```python
from build123d import *

# Parameters (mm, degrees)
CYLINDER004_R           = 5.625
CYLINDER004_DEPTH       = 20
ARRAY_COUNT             = 5
ARRAY_PLACEMENT_ANGLE   = 127.662
CYLINDER003_R           = 1.5
CYLINDER003_DEPTH       = 20
CYLINDER003_PITCH_ANGLE = 90
CYLINDER002_R           = 2.75
CYLINDER002_DEPTH       = 12
BOX_W                   = 3.25
BOX_H                   = 12
BOX_DEPTH               = 12
CYLINDER005_R           = 21.25
CYLINDER005_DEPTH       = 10
TORUS_R                 = 1.5
CYLINDER_R              = 23.75
CYLINDER_DEPTH          = 4
CYLINDER001_R           = 5.5
CYLINDER001_DEPTH       = 8
FILLET_R                = 1


with BuildPart() as array:
    # Cylinder004 → Cylinder004 (new body)
    with BuildSketch(Plane(origin=(13.375, 0, 0), x_dir=(1, 0, 0), z_dir=(0, 0, 1))):
        Circle(CYLINDER004_R)
    extrude(amount=CYLINDER004_DEPTH)

    # Array: Array ×5 about axis
    array_axis = Axis((0, 0, 0), (0, 0, 1))


with BuildPart() as array_1:
    add(array.part)
    for i in range(1, ARRAY_COUNT):
        add(array.part.rotate(array_axis, i * 360 / ARRAY_COUNT))


with BuildPart() as array_2:
    # Array placement: moved
    add(array_1.part.rotate(Axis((0, 0, 0), (0, 0, 1)), ARRAY_PLACEMENT_ANGLE))


with BuildPart() as setscrew:
    # Cylinder003 → Cylinder003 (new body)
    with BuildSketch(Plane.XY):
        Circle(CYLINDER003_R)
    extrude(amount=CYLINDER003_DEPTH)


with BuildPart() as setscrew_1:
    # Cylinder003 pitch: moved
    add(setscrew.part.rotate(Axis((0, 0, 0), (0, 1, 0)), CYLINDER003_PITCH_ANGLE))


with BuildPart() as setscrew_2:
    # Cylinder003 placement: moved
    add(setscrew_1.part.moved(Location((-10, 0, 15))))


with BuildPart() as cylinder001:
    # Cylinder002 → Cylinder002 (new body)
    with BuildSketch(Plane.XY):
        Circle(CYLINDER002_R)
    extrude(amount=CYLINDER002_DEPTH)


with BuildPart() as shaft:
    # Box → Box (new body)
    with BuildSketch(Plane(origin=(-1.6125, -6, 0), x_dir=(1, 0, 0), z_dir=(0, 0, 1))):
        with Locations((1.625, 6)):
            Rectangle(BOX_W, BOX_H)
    extrude(amount=BOX_DEPTH)

    # Common: intersect Cylinder001
    add(cylinder001.part, mode=Mode.INTERSECT)


with BuildPart() as cylinder002:
    # Cylinder005 → Cylinder005 (new body)
    with BuildSketch(Plane.XY.offset(2.1)):
        Circle(CYLINDER005_R)
    extrude(amount=CYLINDER005_DEPTH)


with BuildPart() as torus:
    # Torus → Torus (revolve)
    with BuildSketch(Plane(origin=(0, 0, 2), x_dir=(1, 0, 0), z_dir=(0, -1, 0))):
        with Locations((23.75, 0)):
            Circle(TORUS_R)
    revolve(axis=Axis((0, 0, 2), (0, 0, 1)))


with BuildPart() as cut002:
    # Cylinder → Cylinder (new body)
    with BuildSketch(Plane.XY):
        Circle(CYLINDER_R)
    extrude(amount=CYLINDER_DEPTH)

    # Cut: cut Torus
    add(torus.part, mode=Mode.SUBTRACT)

    # Cut002: cut Cylinder002
    add(cylinder002.part, mode=Mode.SUBTRACT)


with BuildPart() as fillet_body:
    # Cylinder001 → Cylinder001 (new body)
    with BuildSketch(Plane.XY):
        Circle(CYLINDER001_R)
    extrude(amount=CYLINDER001_DEPTH)

    # Fusion: union Cut002
    add(cut002.part)

    # Cut003: cut shaft
    add(shaft.part, mode=Mode.SUBTRACT)

    # Cut004: cut setscrew
    add(setscrew_2.part, mode=Mode.SUBTRACT)

    # Cut005: cut Array
    add(array_2.part, mode=Mode.SUBTRACT)

    # Fillet
    fillet_edges = [fillet_body.edges().sort_by_distance(p)[0] for p in [
        (-21.25, 0, 2.1),
        (-5.5, 0, 2.1),
        (-5.5, 0, 8),
    ]]
    fillet(fillet_edges, radius=FILLET_R)


solid = fillet_body.part
```
Geometry: final body of the model. Coordinates: model frame, mm. A direction names the side the tool comes from. Coordinates: 2 decimals unless noted, no trailing zeros. Order: outer loops, then holes, each group sorted by start corner. A loop starts at its lowest first (then second) coordinate and runs counter-clockwise, first axis right, second up. Notation, with made-up numbers: (57, 35.25) - (93, 35.25) arc R23 cw to (93, 71.25) - close; hole circle Ø9 at (70, 37). An arc over 180 degrees is marked (long way). Write each question's results on one line, items separated by ' | '.
(1) First-contact query: pin 1 Ø4 at (x, z) = (-11.5, 5.5) entering from +Y; pin 2 Ø2 at (y, z) = (9, 4.5) entering from +X; pin 3 Ø4 at (x, z) = (17, 4) entering from -Y. Flat tips, straight axial feed; report the tip coordinate or a pass-through.
Values found:
pin 1: stops at y = 21.46 | pin 2: stops at x = 22.31 | pin 3: stops at y = -18.41
(2) Line query: line 1 (Y direction, x = 0, z = 3.6); line 2 (Y direction, x = 4, z = 2.5); line 3 (X direction, y = 15, z = 1.75). Output: solid intervals per line, ascending. Write a range as [from, to].
Values found:
line 1: y = [-23.75, -21.25], [-5.5, -2.75], [2.75, 5.5], [21.25, 23.75] | line 2: y = [-21.97, -20.67], [-4.06, 4.06], [20.67, 21.97] | line 3: x = [-16.46, -11.66], [-4.68, 3.55], [11.54, 16.46]
(3) Section query A-A, the plane y = 0. Count the separate pieces of the cut face and the enclosed holes in it, plus the area to 3 significant figures.
Values found:
separate pieces: 4 | enclosed holes: 0 | area: 110 mm²
(4) Set-up query: faces 1 (the face through (2, 0, 8)), 2 (the face through (-0.01, -2.75, 3.94)), 3 (the face through (-5, 5, 2.1)). Return all of +Z, -Z, +X, -X, +Y, -Y with unobstructed straight access to the full face (end or side cutting, diameter ignored); none if empty.
Values found:
face 1: +Z, +X, -X, +Y, -Y | face 2: +Z, -Z | face 3: +Z
(5) Section query C-C, the plane z = 5.25. Return the cut outline in (x, y).
Values found:
outline: circle Ø11 at (0, 0); hole (-1.61, -2.23) arc R2.75 ccw to (1.64, -2.21) - (1.64, 2.21) arc R2.75 ccw to (-1.61, 2.23) - close
(6) Mould query, pull axis X, two halves, no side actions, for faces 4 (the face through (5, 0, 0)), 5 (the face through (0.472, -7.745, 1.035)), 6 (the face through (-5.149, -23.185, 3.746)). Classes: +X half, -X half, draft (parallel to the pull), parting line (faces both ways), or undercut.
Values found:
face 4: draft | face 5: undercut | face 6: parting line
